```python
from build123d import *

# Parameters (mm, degrees)
CHAMFER_1_SIZE = 0.655190236
CHAMFER_2_SIZE = 0.5


with BuildPart() as part:
    # ｽｹｯﾁ1 → 回転1 (revolve)
    with BuildSketch(Plane.XY):
        with BuildLine():
            Line((5.7, 0), (5.7, 8))
            Line((5.7, 8), (0, 8))
            Line((0, 8), (0, 10.23))
            ThreePointArc((0, 10.23), (8.046628176, 9.796243245), (16, 8.5))
            Line((16, 8.5), (16, 7))
            Line((16, 7), (8, 7))
            Line((8, 7), (8, 0))
            Line((8, 0), (5.7, 0))
        make_face()
    revolve(axis=Axis((0, 8, 0), (0, 1, 0)))

    # 面取り1
    # the kernel refuses this chamfer: 0.655190236, 0.5 mm, written as the material it takes off along each edge
    with BuildSketch(Plane(origin=(0, 8.5, 0), x_dir=(1, 0, 0), z_dir=(0, 0, 1))) as chamfer_1_piece_1:
        with BuildLine():
            Line((15.512821873, 0.104900382), (16, -CHAMFER_1_SIZE))
            Line((16, -CHAMFER_1_SIZE), (16, 0))
            ThreePointArc((16, 0), (15.747471206, 0.054798761), (15.512821873, 0.104900382))
        make_face()
    revolve(axis=Axis((0, 8.5, 0), (0, 1, 0)), mode=Mode.SUBTRACT)

    # 面取り2
    chamfer_2_edges = [part.edges().sort_by_distance(p)[0] for p in [
        (-5.7, 0, 0),
        (-8, 0, 0),
    ]]
    chamfer(chamfer_2_edges, length=CHAMFER_2_SIZE)


solid = part.part
```
For this review, take the finished solid that the model builds, in its own axes (mm). A direction names the side the tool comes from. Round coordinates to 2 decimals unless told otherwise and drop trailing zeros. Write each loop counter-clockwise with the first axis right and the second up, starting at its lowest first coordinate (ties: lowest second). Pieces come first, ordered by that corner, then holes. Notation, with made-up numbers: (7, 62) -> (45, 62) arc R24 ccw to (45, 73) -> close; hole circle Ø5 at (70.5, -11.5). An arc over 180 degrees is marked (long way). Use one line per item in the form item = value.
Q1. Machinability: for faces 1 (the cylindrical face through (-4.5, 4.3, 3.5)), 2 (the cylindrical face through (-3.47, 7.42, 15.62)), which of the approach directions +Z, -Z, +X, -X, +Y, -Y give a long, thin tool a straight path to every point of the face, cutting with its end or side? Answer none if there is none.
Resolved:
face_1 = -Y
face_2 = +Y, -Y
Q2. To check wall thickness, follow probe 1 along Z at (x, y) = (0, 5.25); probe 2 along X at (y, z) = (4.5, -2). State the ranges of each line that lie inside material, in increasing order. Write a range as from..to.
Resolved:
probe_1 = -8..-5.7, 5.7..8
probe_2 = -7.75..-5.34, 5.34..7.75
Q3. The part is to be moulded in two halves that separate along Z. For faces 3 (the flat face through (-3, 0, -6)), 4 (the cylindrical face through (-1.73, 3.7, 7.81)), 5 (the flat face through (0, 8, 0)), say which applies: released by +Z, released by -Z, zero draft, split by the parting line, or undercut.
Resolved:
face_3 = zero draft
face_4 = split by the parting line
face_5 = undercut
Q4. Consider section A-A (z = 0). State the section outline as (x, y) points.
Resolved:
outline = (-16, 7) -> (-8, 7) -> (-8, 0.5) -> (-7.5, 0) -> (-6.2, 0) -> (-5.7, 0.5) -> (-5.7, 8) -> (5.7, 8) -> (5.7, 0.5) -> (6.2, 0) -> (7.5, 0) -> (8, 0.5) -> (8, 7) -> (16, 7) -> (16, 7.84) -> (15.51, 8.6) arc R74.85 ccw to (-15.51, 8.6) -> (-16, 7.84) -> close
Q5. Consider section B-B (x = 0). State the section outline as (y, z) points, then the cut area to 3 significant figures.
Resolved:
outline = (0, -7.5) -> (0.5, -8) -> (7, -8) -> (7, -16) -> (7.84, -16) -> (8.6, -15.51) arc R74.85 ccw to (8.6, 15.51) -> (7.84, 16) -> (7, 16) -> (7, 8) -> (0.5, 8) -> (0, 7.5) -> (0, 6.2) -> (0.5, 5.7) -> (8, 5.7) -> (8, -5.7) -> (0.5, -5.7) -> (0, -6.2) -> close
area = 105 mm²
Q6. Clearance check with flat-ended pins moving along their axes: pin 1 Ø10 at (x, z) = (-9.5, 3) entering from +Y; pin 2 Ø4 at (x, y) = (-11, 7) entering from +Z; pin 3 Ø3.5 at (x, z) = (1.5, -0.5) entering from -Y. State where each tip first meets the part, or that it passes through.
Resolved:
pin_1 = 10.07
pin_2 = 13.23
pin_3 = 8
Q7. Consider section C-C (y = 4). State the section outline as (x, z) points, then the cut area to 3 significant figures.
Resolved:
outline = circle Ø16 at (0, 0); hole circle Ø11.4 at (0, 0)
area = 99.0 mm²
